from build123d import *

# Parameters (mm, degrees)
SKETCH1_R                = 38.1
BOSS_EXTRUDE1_DEPTH      = 6.35
BOSS_EXTRUDE2_DEPTH      = 12.7
CUT_REVOLVE1_OUTLINE_R   = 4.7625
CUT_REVOLVE1_START       = -1.5875
CUT_REVOLVE1_2_OUTLINE_W = 11
CUT_REVOLVE1_2_OUTLINE_H = 11
CUT_REVOLVE1_2_DEPTH     = 1.5875
CUT_EXTRUDE2_REACH       = 59.15
SKETCH5_R                = 1.5875
CUT_EXTRUDE3_REACH       = 57.358
SKETCH6_R                = 1.5875


with BuildPart() as part:
    # Sketch1 → Boss-Extrude1 (new body)
    with BuildSketch(Plane(origin=(0, 0, 0), x_dir=(1, 0, 0), z_dir=(0, 1, 0))):
        with Locations(Location((0, 0, 0), (0, 0, 270))):
            Circle(SKETCH1_R)
    extrude(amount=BOSS_EXTRUDE1_DEPTH)

    # Sketch2 → Boss-Extrude2 (add)
    with BuildSketch(Plane(origin=(0, 6.35, 0), x_dir=(1, 0, 0), z_dir=(0, 1, 0))):
        with BuildLine():
            ThreePointArc((9.861005618, 36.801773982), (-26.940768363, 26.940768363), (-36.801773982, -9.861005618))
            Line((-36.801773982, -9.861005618), (-24.534515988, -6.574003746))
            ThreePointArc((-24.534515988, -6.574003746), (-17.960512242, 17.960512242), (6.574003746, 24.534515988))
            Line((6.574003746, 24.534515988), (9.861005618, 36.801773982))
        make_face()
    extrude(amount=BOSS_EXTRUDE2_DEPTH)

    # Cut-Revolve1: read off the stored shape, not the designer's step
    # Cut-Revolve1 outline → Cut-Revolve1 (revolve, cut)
    with BuildSketch(Plane.XY):
        with Locations((31.75, 12.7)):
            Circle(CUT_REVOLVE1_OUTLINE_R)
    revolve(axis=Axis((0, 0, 0), (0, 1, 0)), mode=Mode.SUBTRACT)

    # Cut-Revolve1 2 outline → Cut-Revolve1 2 (add)
    with BuildSketch(Plane(origin=(0, 0, 0), x_dir=(0, 1, 0), z_dir=(0.9659258262890682, 0, 0.2588190451025211)).offset(CUT_REVOLVE1_START)):
        with Locations((12.5, -31.5)):
            Rectangle(CUT_REVOLVE1_2_OUTLINE_W, CUT_REVOLVE1_2_OUTLINE_H)
    extrude(amount=CUT_REVOLVE1_2_DEPTH)

    # Sketch5 → Cut-Extrude2 (cut, up to next)
    with BuildSketch(Plane(origin=(0, 0, 0), x_dir=(0.25881904510252135, 0, -0.9659258262890682), z_dir=(0.9659258262890681, 0, 0.2588190451025213)), mode=Mode.PRIVATE) as cut_extrude2_sk1:
        with Locations((31.75, 12.7)):
            Circle(SKETCH5_R)
    cut_extrude2_tool1 = extrude(cut_extrude2_sk1.sketch, amount=-CUT_EXTRUDE2_REACH, mode=Mode.PRIVATE) & part.part
    add(cut_extrude2_tool1.solids().sort_by_distance((8.217505, 12.7, -30.668145))[0], mode=Mode.SUBTRACT)

    # Sketch6 → Cut-Extrude3 (cut, up to next)
    with BuildSketch(Plane(origin=(0, 6.35, 0), x_dir=(1, 0, 0), z_dir=(0, 1, 0)), mode=Mode.PRIVATE) as cut_extrude3_sk1:
        with Locations(Location((0, 0, 0), (0, 0, 270))):
            Circle(SKETCH6_R)
    cut_extrude3_tool1 = extrude(cut_extrude3_sk1.sketch, amount=-CUT_EXTRUDE3_REACH, mode=Mode.PRIVATE) & part.part
    add(cut_extrude3_tool1.solids().sort_by_distance((0, 6.35, 0))[0], mode=Mode.SUBTRACT)


solid = part.part
The listing builds one solid part. Answer for the finished solid, in the listing's coordinates (mm). A direction names the side the tool comes from. Round coordinates to 2 decimals unless told otherwise and drop trailing zeros. Write each loop counter-clockwise with the first axis right and the second up, starting at its lowest first coordinate (ties: lowest second). Pieces come first, ordered by that corner, then holes. Notation, with made-up numbers: M 8,65.25 L 42,65.25 A11 ccw 42,82.25 Z; hole C -30.5,86 d2. An arc over 180 degrees is marked long. Write each question's results on one line, items separated by ' | '. Start each with the question number.
Item 1: Straight lines are drawn through the part: L1, parallel to X at y = 2.5, z = 0; L2, parallel to Y at x = 4, z = -12; L3, parallel to Y at x = -32, z = -3. For each, find the intervals that lie inside material, in ascending order. Write a range as [from, to].
Item 2: A cutting plane is placed at D-D on x = 29. Write down the section's boundary in (y, z), and give its area (3 significant figures).
Item 3: A cutting plane is placed at C-C on y = 15.5. Write down the section's boundary in (x, z), and give its area (3 significant figures).
Item 4: Flat-ended cylindrical pins translate along their axes: pin 1 Ø4 at (x, z) = (-28.5, 26) entering from +Y; pin 2 Ø2 at (x, y) = (29, 3.5) entering from +Z; pin 3 Ø8 at (y, z) = (9.5, 9.5) entering from -X. Find the tip coordinate at first contact, or state that the pin passes through.
Item 5: A cutting plane is placed at A-A on x = 0. State how many separate pieces and enclosed holes the cut face has, and give its area (3 significant figures).
Item 6: For faces 1 (the face through (7.2, 12.6, -33)), 2 (the face through (-20, 19.05, -20)), determine the directions among +Z, -Z, +X, -X, +Y, -Y from which every point of the face is accessible in a straight line to the end or side of a thin tool.
Item 7: For a pull along Z with two mould halves and no side action, classify faces 3 (the face through (-18.22, 12.61, -17.7)), 4 (the face through (-26.665, 15.433, 7.145)), 5 (the face through (1, 0, 8)) as pulls with the +Z half, pulls with the -Z half, needs draft (parallel to the pull), parting line crosses it, or undercut.
Check sheet entries:
1) L1: [-38.1, -1.59], [1.59, 38.1] | L2: [0, 6.35] | L3: [0, 7.95], [17.45, 19.05]
2) outline: M 0,-24.71 L 6.35,-24.71 L 6.35,24.71 L 0,24.71 Z | area: 314 mm²
3) outline: M -36.8,9.86 A38.1 ccw 9.86,-36.8 L 6.57,-24.53 A25.4 cw -24.53,6.57 L -26.95,7.22 A27.9 ccw 5.68,-27.31 L 7.67,-34.77 A35.6 cw -34.39,9.21 Z | area: 344 mm²
4) pin 1: y = 6.35 | pin 2: z = 25.84 | pin 3: x = -37.7
5) separate pieces: 2 | enclosed holes: 1 | area: 554 mm²
6) face 1: none | face 2: +Z, -Z, +X, -X, +Y
7) face 3: undercut | face 4: pulls with the +Z half | face 5: needs draft
